Build history of the part. All positions in model axes, mm. Face numbers are marked on the shaded views. Give positions to 0.01 mm unless a question says otherwise; leave off trailing zeros. Write each loop counter-clockwise with the first axis right and the second up, starting at its lowest first coordinate (ties: lowest second). Pieces come first, ordered by that corner, then holes. Notation, with made-up numbers: (36, 25.5) -> (72, 25.5) arc R9 ccw to (72, 42.5) -> close; hole circle Ø4 at (42.5, -27). An arc over 180 degrees is marked (long way). One line per question, with ' | ' between items. Start each with the question number.
(1) Pin check, flat tips, straight feed: P1, Ø10.5, axis at x = 0, z = 0, coming from the -Y side; P2, Ø1.5, axis at y = 1, z = -7, coming from the -X side; P3, Ø1, axis at x = -5.5, y = 5, coming from the -Z side; P4, Ø3, axis at y = 5, z = -2, coming from the -X side. Stop position of each tip, or through.
(2) Pull direction Z, two halves, no side cores. Call the marked faces 1, 2 and 3: released by +Z, released by -Z, zero draft, split by the parting line, or undercut.
(3) Drill centre lines: probe 1 along X at (y, z) = (8, 0); probe 2 along Y at (x, z) = (-6.5, -7.25); probe 3 along X at (y, z) = (6.5, 3.25). Where is each one in solid material? Low to high. Write a range as from..to.
(4) Band-saw the part on B-B, the plane x = 0. Give the cut face in (y, z), and give its area (3 significant figures).
(5) Band-saw the part on C-C, the plane y = 3. Give the cut face in (x, z), and give its area (3 significant figures).
(6) Band-saw the part on A-A, the plane z = 0. Give the cut face in (x, y).
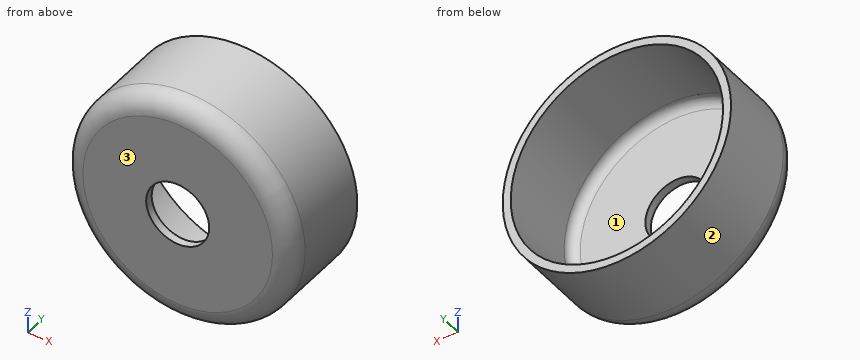
from build123d import *


with BuildPart() as part:
    # Sketch1 → Revolve1 (revolve)
    with BuildSketch(Plane.XY, mode=Mode.PRIVATE) as revolve1_sk:
        with BuildLine():
            Line((3.302, 0), (9.9314, 0))
            ThreePointArc((9.9314, 0), (11.368240979, 0.595159021), (11.9634, 2.032))
            Line((11.9634, 2.032), (11.9634, 10))
            Line((11.9634, 10), (11.1252, 10))
            Line((11.1252, 10), (11.1252, 1.8382))
            ThreePointArc((11.1252, 1.8382), (10.832306781, 1.131093219), (10.1252, 0.8382))
            Line((10.1252, 0.8382), (3.302, 0.8382))
            Line((3.302, 0.8382), (3.302, 0))
        make_face()
    revolve(revolve1_sk.sketch.rotate(Axis((0, 0, 0), (0, 1, 0)), 90), axis=Axis((0, 0, 0), (0, 1, 0)))  # turned: the seam where the file's is


solid = part.part
Results:
1) P1: stops at y = 0 | P2: stops at x = -10.01 | P3: stops at z = -10.87 | P4: stops at x = -11.95
2) face 1: undercut | face 2: split by the parting line | face 3: zero draft
3) probe 1: x = -11.96..-11.13, 11.13..11.96 | probe 2: y = 0..0.84 | probe 3: x = -11.51..-10.64, 10.64..11.51
4) outline: (0, -9.93) arc R2.03 ccw to (2.03, -11.96) -> (10, -11.96) -> (10, -11.13) -> (1.84, -11.13) arc R1 cw to (0.84, -10.13) -> (0.84, -3.3) -> (0, -3.3) -> close; (0, 3.3) -> (0.84, 3.3) -> (0.84, 10.13) arc R1 cw to (1.84, 11.13) -> (10, 11.13) -> (10, 11.96) -> (2.03, 11.96) arc R2.03 ccw to (0, 9.93) -> close | area: 28.5 mm²
5) outline: circle Ø23.93 at (0, 0); hole circle Ø22.25 at (0, 0) | area: 60.8 mm²
6) outline: (-11.96, 2.03) arc R2.03 ccw to (-9.93, 0) -> (-3.3, 0) -> (-3.3, 0.84) -> (-10.13, 0.84) arc R1 cw to (-11.13, 1.84) -> (-11.13, 10) -> (-11.96, 10) -> close; (3.3, 0) -> (9.93, 0) arc R2.03 ccw to (11.96, 2.03) -> (11.96, 10) -> (11.13, 10) -> (11.13, 1.84) arc R1 cw to (10.13, 0.84) -> (3.3, 0.84) -> close
